Source: CAD feature listing. Evaluate the final solid. Frame: model axes, mm. A direction names the side the tool comes from. Coordinates: 2 decimals unless noted, no trailing zeros. Order: outer loops, then holes, each group sorted by start corner. A loop starts at its lowest first (then second) coordinate and runs counter-clockwise, first axis right, second up. Notation, with made-up numbers: (-5, 6) -> (2, 6) arc R18 cw to (2, 35) -> close; hole circle Ø11 at (80.5, -38.75). An arc over 180 degrees is marked (long way). Write item = value, one per line. Start each with the question number.
Item 1: Set-up query: faces 1 (the flat face through (-4, -0.75, 0)), 2 (the cylindrical face through (-0.08, 11.18, -2.4)). Return all of +Z, -Z, +X, -X, +Y, -Y with unobstructed straight access to the full face (end or side cutting, diameter ignored); none if empty.
Item 2: Ray query, line 1 along X through (y, z) = (-1, 0); line 2 along Z through (x, y) = (0, -1.5); line 3 along Z through (x, y) = (-1, -2). Return the intervals inside material, ascending. Write a range as [from, to].
Item 3: Section query D-D (x = 0). Output: boundary loops of the cut face in (y, z), then the cut area to 3 significant figures.
Item 4: Section query A-A (z = 0). Output: boundary loops of the cut face in (x, y), then the cut area to 4 significant figures.
Item 5: Section query C-C (x = 3.5). Output: boundary loops of the cut face in (y, z), then the cut area to 3 significant figures.
Item 6: Mould query, pull axis X, two halves, no side actions, for faces 3 (the flat face through (-2.544, -7.518, 1.996)), 4 (the flat face through (-5.5, 1, 0)), 5 (the flat face through (5, -8.75, -1)). Classes: released by +X, released by -X, zero draft, split by the parting line, or undercut.
Item 7: Section query B-B (y = -3). Output: boundary loops of the cut face in (x, z).
Autodesk Inventor part; units mm, degrees
ref_plane "plane_support" through (-5.5, -7.5, -3) normal (0, -1, 0) x (1, 0, 0)
ref_plane "plane_support_frontb" through (-2.75, 0, 0) normal (1, 0, 0) x (0, 0, -1)
ref_plane "plane_support_frontt" through (2.75, 0, 0) normal (-1, 0, 0) x (0, 0, 1)
sketch "Sketch14" plane through (0, 0, 0) normal (1, 0, 0) x (0, 1, 0)
  line L0 (-12.85, 0) -> (15.85, 0)
  line L1 (0, -4.2) -> (0, 4.2)
  line L2 (8.75, -3) -> (-8.75, -3)
  line L3 (-8.75, -3) -> (-8.75, 3)
  line L4 (-8.75, 3) -> (8.75, 3)
  line L5 (8.75, 3) -> (8.75, -3) construction
  line L6 (8.75, -3) -> (-8.75, 3) construction
  line L7 (-8.75, -3) -> (8.75, 3) construction
  line L8 (5.25, 3) -> (5.25, -3) construction
  line L9 (-6.25, 3) -> (-6.25, -3) construction
  arc A0 (8.75, -3) -> (8.75, 3) centre (8.75, 0) ccw
  circle A1 centre (8.75, 0) radius 1.25 construction
  circle A2 centre (8.75, 0) radius 3 construction
  line L10 (5.75, 3) -> (5.75, -3) construction
  line L11 (11.75, 3) -> (11.75, -3)
  line L12 (11.75, -3) -> (8.75, -3)
  line L13 (8.75, 3) -> (11.75, 3)
  point P0 (0, 0)
  point P1 (0, 0)
  dimension "d72" = 6
  dimension "d74" = 2.5
  dimension "d75" = 2.5
  dimension "d76" = 0.5
  dimension "d105" = 18
extrude "ext_main" add sketch "Sketch14" along normal mid plane 11
sketch "sk_channel_nut" plane through (-5.5, -8.75, -3) normal (0, -1, 0) x (1, 0, 0)
  line L0 (-2.2, 3) -> (13.2, 3)
  line L1 (5.5, -1.8497) -> (5.5, 7.8497)
  circle A0 centre (5.5, 3) radius 2
  line L2 (5.5, 6.4641) -> (2.5, 4.7321)
  line L3 (2.5, 4.7321) -> (2.5, 1.2679)
  line L4 (2.5, 1.2679) -> (5.5, -0.4641)
  line L5 (5.5, -0.4641) -> (8.5, 1.2679)
  line L6 (8.5, 1.2679) -> (8.5, 4.7321)
  line L7 (8.5, 4.7321) -> (5.5, 6.4641)
  circle A1 centre (1.5, 3) radius 1
  circle A2 centre (9.5, 3) radius 1
  line L8 (1.5, 4) -> (2.5, 4)
  line L9 (1.5, 2) -> (2.5, 2)
  line L10 (9.5, 4) -> (8.5, 4)
  line L11 (9.5, 2) -> (8.5, 2)
  line L12 (0, 0) -> (11, 0)
  line L13 (0, 6) -> (11, 6)
  line L14 (0, 0) -> (0, 6)
  line L15 (3.4, 6) -> (3.4, 5.2517)
  line L16 (3.4456, 0.722) -> (3.4456, 0)
  line L17 (7.5544, 0.722) -> (7.5544, 0)
  line L18 (7.6, 6) -> (7.6, 5.2517)
  point P0 (2.5, 3)
  dimension "d85" = 4
  dimension "d86" = 120
  dimension "d87" = 6
  dimension "d88" = 2
  dimension "d95" = 4.2
extrude "ext_cut_channel" cut sketch "sk_channel_nut" against normal through all contours A0 L1 L0 | L0 L1 A0 | L1 A0 L0 | L0 A0 L1
extrude "ext_cut_bottomscrews" cut sketch "sk_channel_nut" against normal blind 8 contours A1 L0 | L0 A1 | A1 L8 L3 | L3 L9 A1 | A2 L0 | A2 L11 L6 | L6 L10 A2 | L0 A2
extrude "ext_cut_bottom_nut" cut sketch "sk_channel_nut" against normal blind 2.5 contours L3 L2 L13 L1 A0 L0 | L0 A0 L1 L12 L4 L3 | L16 L4 L12 | L13 L2 L15 | A0 L1 L0 | L0 L1 A0 | L12 L1 L4 | L2 L1 L13 | L1 A0 L0 | L0 A0 L1 | L1 L13 L7 L6 L0 A0 | A0 L0 L6 L5 L12 L1 | L1 L12 L5 | L7 L13 L1 | L5 L17 L12 | L13 L18 L7
fillet "Fillet1" radius 2 1 edges at (0, 11.75, -3)
sketch "Sketch19" plane through (-5.5, -7.5, -3) normal (0, -1, 0) x (1, 0, 0)
  line L0 (3.4, 6) -> (7.6, 6)
  line L1 (3.4, 5.2517) -> (3.4, 6)
  line L2 (2.5, 4.7321) -> (3.4, 5.2517)
  line L3 (2.5, 4) -> (2.5, 4.7321)
  line L4 (2.5, 2) -> (2.5, 4)
  line L5 (2.5, 1.2679) -> (2.5, 2)
  line L6 (3.4456, 0.722) -> (2.5, 1.2679)
  line L7 (3.4456, 0) -> (3.4456, 0.722)
  line L8 (7.5544, 0) -> (3.4456, 0)
  line L9 (7.5544, 0.722) -> (7.5544, 0)
  line L10 (8.5, 1.2679) -> (7.5544, 0.722)
  line L11 (8.5, 2) -> (8.5, 1.2679)
  line L12 (8.5, 4) -> (8.5, 2)
  line L13 (8.5, 4.7321) -> (8.5, 4)
  line L14 (7.6, 5.2517) -> (8.5, 4.7321)
  line L15 (7.6, 6) -> (7.6, 5.2517)
  circle A0 centre (5.5, 3) radius 2
  line L16 (3.65, 5.75) -> (7.35, 5.75) construction
  line L17 (7.35, 5.75) -> (7.35, 5.1073)
  line L18 (7.35, 5.1073) -> (8.25, 4.5877)
  line L19 (8.25, 4.5877) -> (8.25, 4)
  line L20 (8.25, 4) -> (8.25, 2)
  line L21 (8.25, 2) -> (8.25, 1.4123)
  line L22 (8.25, 1.4123) -> (7.3044, 0.8664)
  line L23 (7.3044, 0.8664) -> (7.3044, 0.25)
  line L24 (7.3044, 0.25) -> (3.6956, 0.25) construction
  line L25 (3.6956, 0.25) -> (3.6956, 0.8664)
  line L26 (3.6956, 0.8664) -> (2.75, 1.4123)
  line L27 (2.75, 1.4123) -> (2.75, 2)
  line L28 (2.75, 2) -> (2.75, 4)
  line L29 (2.75, 4) -> (2.75, 4.5877)
  line L30 (2.75, 4.5877) -> (3.65, 5.1073)
  line L31 (3.65, 5.1073) -> (3.65, 5.75)
  line L32 (3.65, 5.75) -> (7.35, 5.75)
  line L33 (7.35, 5.75) -> (7.35, 6)
  line L34 (7.35, 6) -> (3.65, 6)
  line L35 (3.65, 6) -> (3.65, 5.75)
  line L36 (3.6956, 0.25) -> (7.3044, 0.25)
  line L37 (7.3044, 0.25) -> (7.3044, 0)
  line L38 (7.3044, 0) -> (3.6956, 0)
  line L39 (3.6956, 0) -> (3.6956, 0.25)
  point P0 (5.5, 3)
  dimension "d97" = 0.25
sketch "Sketch20" plane through (-2.75, 0, 0) normal (1, 0, 0) x (0, 0, -1)
  circle A0 centre (0, 9) radius 1.25
  arc A1 (3, 9) -> (-3, 9) centre (0, 9) ccw
  line L0 (-3, 6) -> (-3, 9)
  line L1 (3, 6) -> (-3, 6)
  line L2 (3, 9) -> (3, 6)
  line L3 (-3, 7) -> (3, 7)
  point P0 (0, 0)
  dimension "d102" = 1
equation "\"d74\" = nut_m3_thickness_max"
equation "\"d75\" = screw_m2_bore_loose"
equation "\"d87\" = nut_m3_width_acrossflats"
equation "\"d88\" = screw_m2_bore_selfthreading"
equation "\"d95\" = 0.7 * nut_m3_width_acrossflats"
equation "\"d89\" = linact_rod_effective_length + nut_m3_thickness_max"
equation "\"d93\" = nut_m3_thickness_max"
equation "\"d97\" = print_support_z_clearance"
equation "\"d102\" = print_support_xy_clearance"
equation "\"d96\" = print_support_xy_clearance"
equation "\"d100\" = print_support_z_clearance"
equation "\"d101\" = print_support_z_clearance"
properties part number "empty"
Computed:
q1.face_1 = -Y
q1.face_2 = -Z, +X, -X, +Y
q2.line_1 = [-5.5, -5], [-3, -2], [2, 3], [5, 5.5]
q2.line_2 = [-3, -2], [2, 3]
q2.line_3 = [-3, -1.73], [1.73, 3]
q3.outline = (-6.25, -3) -> (9.75, -3) arc R2 ccw to (11.48, -2) -> (-6.25, -2) -> close; (-6.25, 2) -> (11.75, 2) -> (11.75, 3) -> (-6.25, 3) -> close
q3.area = 35.2 mm^2
q4.outline = (-5.5, -8.75) -> (-5, -8.75) -> (-5, -0.75) -> (-3, -0.75) -> (-3, -6.25) -> (-2, -6.25) -> (-2, 11.75) -> (-5.5, 11.75) -> close; (2, -6.25) -> (3, -6.25) -> (3, -0.75) -> (5, -0.75) -> (5, -8.75) -> (5.5, -8.75) -> (5.5, 11.75) -> (2, 11.75) -> close
q4.area = 106.5 mm^2
q5.outline = (-8.75, -3) -> (9.75, -3) arc R2 ccw to (11.75, -1) -> (11.75, 3) -> (-8.75, 3) -> (-8.75, 1) -> (-0.75, 1) -> (-0.75, -1) -> (-8.75, -1) -> close
q5.area = 106 mm^2
q6.face_3 = undercut
q6.face_4 = released by -X
q6.face_5 = zero draft
q7.outline = (-5.5, -3) -> (5.5, -3) -> (5.5, 3) -> (-5.5, 3) -> close; hole (-4, -1) -> (-3, -1) -> (-3, 1) -> (-4, 1) arc R1 ccw to start; hole circle Ø4 at (0, 0); hole (3, -1) -> (4, -1) arc R1 ccw to (4, 1) -> (3, 1) -> close
